The model under review builds one solid part; all positions refer to its coordinate system, in mm. Round coordinates to 2 decimals unless told otherwise and drop trailing zeros. Write each loop counter-clockwise with the first axis right and the second up, starting at its lowest first coordinate (ties: lowest second). Pieces come first, ordered by that corner, then holes. Notation, with made-up numbers: M 10,1.5 L 52,1.5 A27 ccw 52,20.5 Z; hole C 57.5,-12 d4. An arc over 180 degrees is marked long. One line per item, written item: value. Start each with the question number.
1) Take a section at A-A, the plane x = 21. Write out the cut boundary in (y, z) (3 decimals), and give its area (3 significant figures).
2) For P1, Ø1.5, axis at x = 31.5, y = 13.5, coming from the +Z side; P2, Ø1, axis at x = 16.5, y = -15.5, coming from the +Z side; P3, Ø1.5, axis at x = 20.5, z = 4, coming from the +Y side, all flat-tipped, find the tip position at first contact; note any pin that passes through.
3) Wall thickness on probe 1 along Z at (x, y) = (22, 0) (3 decimals); probe 2 along Z at (x, y) = (17, -5.5); probe 3 along Z at (x, y) = (37, -11.5): over which ranges is each line inside the solid? List them lowest first.
4) Mouldability with a two-part tool opening along Y and no side actions: class faces 1 (the face through (49.99, 0, 4)), 2 (the face through (43.96, -0.69, -3.1)), 3 (the face through (25.311, 21.199, 6.676)) as +Y half, -Y half, draft (parallel to the pull), parting line (faces both ways), or undercut.
from build123d import *

# Parameters (mm, degrees)
F0_R           = 22.225
F1_DEPTH       = 50.8
F2_R           = 19.05
F3_R           = 15.875
F4_DEPTH       = 38.1
F5_R           = 1.27
F6_R           = 3.175
F7_DEPTH       = 50.801
F8_R           = 10.16
F9_W           = 6.6301524639
F9_H           = 19.9486073107
F10_DEPTH      = 22.2260001
F10_DEPTH_BACK = 25.4


with BuildPart() as f1:
    # F0 (on Right) → F1 (new body)
    with BuildSketch(Plane.YZ):
        Circle(F0_R)
    extrude(amount=F1_DEPTH)

    # F2
    f2_edges = [f1.edges().sort_by_distance(p)[0] for p in [
        (0, -22.225, 0),
        (50.8, -22.225, 0),
    ]]
    fillet(f2_edges, radius=F2_R)

    # F3 (on Right) → F4 (cut)
    with BuildSketch(Plane.YZ):
        Circle(F3_R)
    extrude(amount=F4_DEPTH, mode=Mode.SUBTRACT)

    # F5
    f5_edges = [f1.edges().sort_by_distance(p)[0] for p in [
        (4.850968, -15.875, 0),
    ]]
    fillet(f5_edges, radius=F5_R)

    # F6 (on Right) → F7 (cut, through all)
    with BuildSketch(Plane.YZ):
        Circle(F6_R)
    extrude(amount=F7_DEPTH, mode=Mode.SUBTRACT)

    # F8
    f8_edges = [f1.edges().sort_by_distance(p)[0] for p in [
        (38.1, -15.875, 0),
    ]]
    fillet(f8_edges, radius=F8_R)

    # F9 (on Front) → F10 (cut, two sides)
    with BuildSketch(Plane.XZ) as f10_sk:
        with Locations((53.3047877252, -1.149632968)):
            Rectangle(F9_W, F9_H)
    extrude(amount=-F10_DEPTH, mode=Mode.SUBTRACT)
    extrude(f10_sk.sketch, amount=F10_DEPTH_BACK, mode=Mode.SUBTRACT)


solid = f1.part
Checked values:
1. outline: C 0,0 d44.45; hole C 0,0 d31.75
1. area: 760 mm2
2. P1: stops at z = 18.2
2. P2: stops at z = 16.18
2. P3: stops at y = 21.99
3. probe 1: z = -22.225 to -15.875, 15.875 to 22.225
3. probe 2: z = -21.42 to -14.89, 14.89 to 21.42
3. probe 3: z = -18.15 to 18.15
4. face 1: draft
4. face 2: undercut
4. face 3: parting line
